Check sheet for the modelled part. Datum: model origin and axes. Units: mm. A direction names the side the tool comes from. Give positions to 0.01 mm unless a question says otherwise; leave off trailing zeros. Write each loop counter-clockwise with the first axis right and the second up, starting at its lowest first coordinate (ties: lowest second). Pieces come first, ordered by that corner, then holes. Notation, with made-up numbers: M -5,-3 L 25,-3 A25 ccw 25,12 Z; hole C 20.5,33.25 d6. An arc over 180 degrees is marked long. Use CSV: the item, a comma, the result in double quotes. Start each with the question number.
1. Cross-section at A-A, the plane z = 30. Enter the section's corners in (x, y).
2. Mould release check, pull along X, two halves, no side actions. Record for faces 6 (the face through (121.885, -51, 46)), 7 (the face through (79.014, -108, 63)), 8 (the face through (69, 12.7, 64)): +X half, -X half, draft (parallel to the pull), parting line (faces both ways), or undercut.
3. Scan lines: line 1 (X direction, y = -37.5, z = 46); line 2 (Y direction, x = 118, z = 26.5); line 3 (Y direction, x = 75.5, z = 39.5). Record each from-to range of solid material in increasing order.
4. Depth check by flat-ended pin: P1, Ø14.5, axis at x = 107.5, z = 45, coming from the +Y side; P2, Ø10, axis at y = -106.5, z = 73, coming from the +X side; P3, Ø4, axis at y = 7, z = 68.5, coming from the +X side. Enter the tip coordinate at first touch or a pass-through.
5. Access from +Z, -Z, +X, -X, +Y, -Y to the whole of each face (thin tool, end or side, straight path). Record for faces 1 (the face through (28, 0, 36)), 2 (the face through (9.49, -50, 46)), 3 (the face through (66, -101.6, 100)), 4 (the face through (26, -101.6, 36)), 5 (the face through (104, -101.6, 36)).
6. Cross-section at B-B, the plane z = 101. Enter the section's corners in (x, y).
7. Cross-section at D-D, the plane y = -66.5. Enter the section's corners in (x, z).
8. Cross-section at C-C, the plane x = 72. Enter the section's corners in (y, z), and give its area (3 significant figures).
from build123d import *

# Parameters (mm, degrees)
F0_W     = 129.983455
F0_H     = 71.484342
F1_DEPTH = 101.6
F3_DEPTH = 50.8
F4_W     = 25.4
F4_H     = 127
F5_DEPTH = 12.7
F6_W     = 25.4
F6_H     = 127
F7_DEPTH = 12.7


with BuildPart() as f1:
    # F0 (on Front) → F1 (new body)
    with BuildSketch(Plane.XZ):
        with Locations((64.991727, 35.742171)):
            Rectangle(F0_W, F0_H)
    extrude(amount=F1_DEPTH)

    # F2 (on face) → F3 (cut)
    with BuildSketch(Plane.XY.offset(71.484342)):
        Polygon((121.884853, -11.710611), (64.991727, -11.710611), (9.490403, -11.710611), (9.490403, -89.278609), (121.884853, -89.278609), (121.884853, -50.8), align=None)
    extrude(amount=-F3_DEPTH, mode=Mode.SUBTRACT)

    # F4 (on face) → F5 (join)
    with BuildSketch(Plane.XZ.offset(101.6)):
        with Locations((66.31402, 63.5)):
            Rectangle(F4_W, F4_H)
    extrude(amount=F5_DEPTH)

    # F6 (on face) → F7 (join)
    with BuildSketch(Plane(origin=(0, 0, 0), x_dir=(-1, 0, 0), z_dir=(0, 1, 0))):
        with Locations((-69.025247, 63.5)):
            Rectangle(F6_W, F6_H)
    extrude(amount=F7_DEPTH)


solid = f1.part
Worked answers:
1,outline,"M 0,-101.6 L 53.61,-101.6 L 53.61,-114.3 L 79.01,-114.3 L 79.01,-101.6 L 129.98,-101.6 L 129.98,0 L 81.73,0 L 81.73,12.7 L 56.33,12.7 L 56.33,0 L 0,0 Z; hole M 9.49,-89.28 L 121.88,-89.28 L 121.88,-11.71 L 9.49,-11.71 Z"
2,face 6,"undercut"
2,face 7,"+X half"
2,face 8,"draft"
3,line 1,"x = 0 to 9.49, 121.88 to 129.98"
3,line 2,"y = -101.6 to -89.28, -11.71 to 0"
3,line 3,"y = -114.3 to -89.28, -11.71 to 12.7"
4,P1,"stops at y = 0"
4,P2,"stops at x = 79.01"
4,P3,"stops at x = 81.73"
5,face 1,"+Z, -Z, -X, +Y"
5,face 2,"+Z"
5,face 3,"+Z, +X, -X"
5,face 4,"+Z, -Z, -X, -Y"
5,face 5,"+Z, -Z, +X, -Y"
6,outline,"M 53.61,-114.3 L 79.01,-114.3 L 79.01,-101.6 L 53.61,-101.6 Z; M 56.33,0 L 81.73,0 L 81.73,12.7 L 56.33,12.7 Z"
7,outline,"M 0,0 L 129.98,0 L 129.98,71.48 L 121.88,71.48 L 121.88,20.68 L 9.49,20.68 L 9.49,71.48 L 0,71.48 Z"
8,outline,"M -114.3,0 L 12.7,0 L 12.7,127 L 0,127 L 0,71.48 L -11.71,71.48 L -11.71,20.68 L -89.28,20.68 L -89.28,71.48 L -101.6,71.48 L -101.6,127 L -114.3,127 Z"
8,area,"6,550 mm^2"
